Here's the drawing with two shaded views (mm, measured from the low corner). I have some questions. A direction names the side the tool comes from. Round coordinates to 2 decimals unless told otherwise and drop trailing zeros. Loops run counter-clockwise (first coordinate to the right, second up) from the corner with the lowest first, then second, coordinate; pieces in that order, holes last.
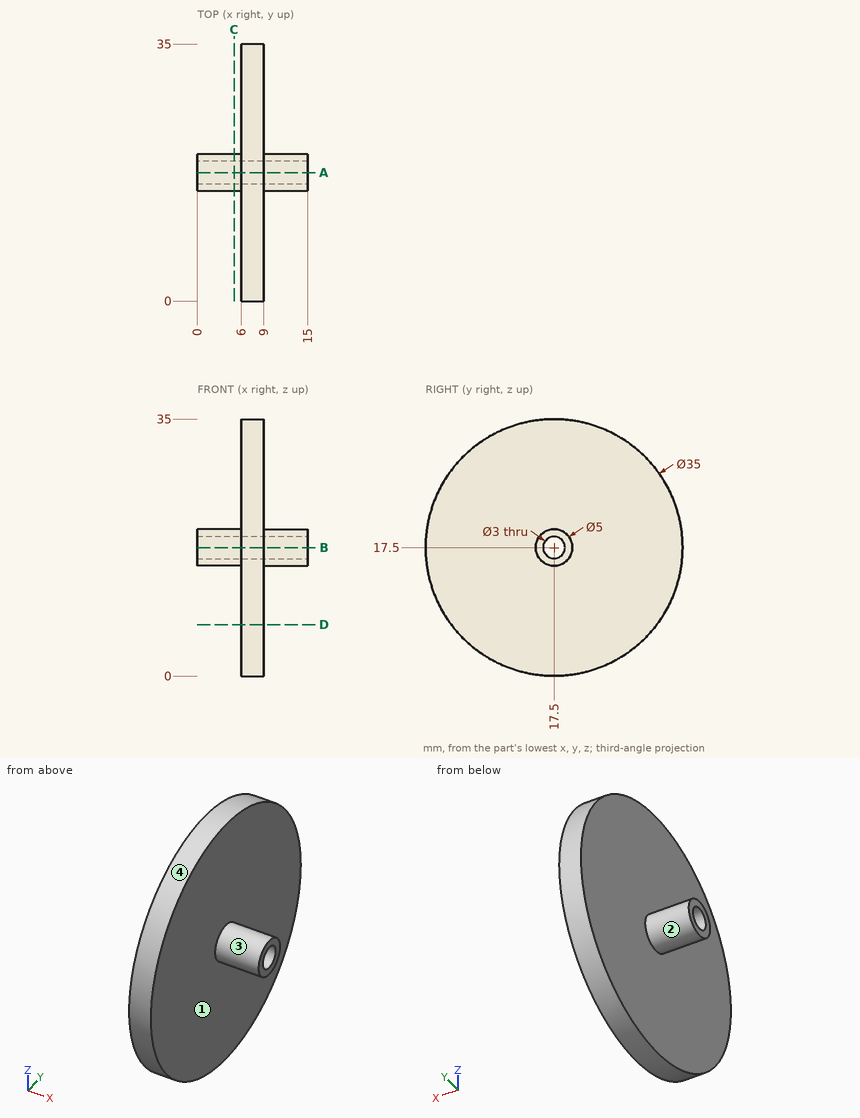
Item 1: If I drill on line 1 along Z through (x, y) = (10, 17.5); line 2 along Z through (x, y) = (7, 17.5); line 3 along X through (y, z) = (22.5, 18.5), over which ranges is the centre line in solid material (lowest first)?
Results list:
line 1: z = 15 to 16, 19 to 20
line 2: z = 0 to 16, 19 to 35
line 3: x = 6 to 9
Item 2: We'd pull the mould along Y, two halves only. Please class the marked faces 1 and 2: released by +Y, released by -Y, zero draft, split by the parting line, or undercut.
Results list:
face 1: zero draft
face 2: split by the parting line
Item 3: For the marked faces 3 and 4, which set-ups out of +Z, -Z, +X, -X, +Y, -Y let a thin tool reach every point of the face, with its end or its side?
Results list:
face 3: +X
face 4: +X, -X
Item 4: Will these pins go through, and if not, where does the flat tip stop? pin 1 (3 mm diameter, centred on x = 5.5, z = 26.5, fed in from -Y); pin 2 (12 mm diameter, centred on y = 6.5, z = 21, fed in from +X); pin 3 (10.5 mm diameter, centred on y = 10.5, z = 21.5, fed in from -X); pin 4 (5 mm diameter, centred on x = 12, y = 27.5, fed in from +Z).
Results list:
pin 1: stops at y = 1.73
pin 2: stops at x = 9
pin 3: stops at x = 6
pin 4: passes through
Item 5: If we section it at D-D, the plane z = 7: Please give me the cut outline in (x, y), then the cut area to 3 significant figures.
Results list:
outline: (6, 3.5) - (9, 3.5) - (9, 31.5) - (6, 31.5) - close
area: 84.0 mm2
Item 6: If we section it at A-A, the plane y = 17.5: Please give me the cut outline in (x, z), then the cut area to 3 significant figures.
Results list:
outline: (0, 15) - (6, 15) - (6, 0) - (9, 0) - (9, 15) - (15, 15) - (15, 16) - (0, 16) - close; (0, 19) - (15, 19) - (15, 20) - (9, 20) - (9, 35) - (6, 35) - (6, 20) - (0, 20) - close
area: 120 mm2
Item 7: If we section it at C-C, the plane x = 5: Please give me the cut outline in (y, z), then the cut area to 3 significant figures.
Results list:
outline: circle Ø5 at (17.5, 17.5); hole circle Ø3 at (17.5, 17.5)
area: 12.6 mm2
